```python
from build123d import *

# Parameters (mm, degrees)
SKETCH1_R           = 9.525
BOSS_EXTRUDE1_DEPTH = 3.175
SKETCH3_R           = 0.508
CUT_EXTRUDE1_DEPTH  = 25.4
SKETCH6_W           = 1.016
SKETCH6_H           = 1.016
CUT_EXTRUDE2_DEPTH  = 7.366
SKETCH7_W           = 1.012612731
SKETCH7_H           = 1.016
CUT_EXTRUDE3_DEPTH  = 7.366
SKETCH4_R           = 0.508


with BuildPart() as part:
    # Sketch1 → Boss-Extrude1 (new body)
    with BuildSketch(Plane(origin=(0, 0, 0), x_dir=(1, 0, 0), z_dir=(0, 1, 0))):
        Circle(SKETCH1_R)
    extrude(amount=BOSS_EXTRUDE1_DEPTH)

    # Sketch3 → Cut-Extrude1 (cut, symmetric)
    with BuildSketch(Plane.XY):
        with Locations((-8.509, 1.5875)):
            Circle(SKETCH3_R)
    extrude(amount=CUT_EXTRUDE1_DEPTH, both=True, mode=Mode.SUBTRACT)

    # Sketch6 → Cut-Extrude2 (cut)
    with BuildSketch(Plane.XY.offset(-7.62)):
        with Locations((-9.017, 1.5875)):
            Rectangle(SKETCH6_W, SKETCH6_H)
    extrude(amount=CUT_EXTRUDE2_DEPTH, mode=Mode.SUBTRACT)

    # Sketch7 → Cut-Extrude3 (cut)
    with BuildSketch(Plane.XY.offset(7.62)):
        with Locations((-9.015306366, 1.5875)):
            Rectangle(SKETCH7_W, SKETCH7_H)
    extrude(amount=-CUT_EXTRUDE3_DEPTH, mode=Mode.SUBTRACT)

    # Cut-Sweep1: sweep along a path in Sketch5
    with BuildLine(Plane(origin=(0, 0, 0), x_dir=(1, 0, 0), z_dir=(0, 1, 0))) as cut_sweep1_path:
        ThreePointArc((-7.554809844, -0.994609585), (7.62, 0), (-7.554809844, 0.994609585))
    # Sketch4 → Cut-Sweep1 (sweep, cut)
    with BuildSketch(Plane.XY):
        with Locations((9.525, 1.5875)):
            Circle(SKETCH4_R)
    sweep(path=cut_sweep1_path.line, mode=Mode.SUBTRACT)


solid = part.part
```
The model under review builds one solid part; all positions refer to its coordinate system, in mm. A direction names the side the tool comes from. Round coordinates to 2 decimals unless told otherwise and drop trailing zeros. Loops run counter-clockwise (first coordinate to the right, second up) from the corner with the lowest first, then second, coordinate; pieces in that order, holes last. Notation, with made-up numbers: M 61,24 L 95,24 A20 ccw 95,43 Z; hole C -12.5,-35 d5. An arc over 180 degrees is marked long. Put each result on its own line as item: value.
Q1. Consider section B-B, the plane y = 2.4. Give the boundary of the cut face in (x, z) (3 decimals), then the cut area to 3 significant figures.
Result set:
outline: C 0,0 d19.05
area: 285 mm²
Q2. Machinability: for faces 4 (the flat face through (-9, 2.096, -2)), 5 (the cylindrical face through (-8.04, 1.39, 0.06)), 6 (the flat face through (-9, 1.08, 2)), which of the approach directions +Z, -Z, +X, -X, +Y, -Y give a long, thin tool a straight path to every point of the face, cutting with its end or side? Answer none if there is none.
Result set:
face 4: -Z, -X
face 5: +Z, -Z
face 6: +Z, -X
Q3. Mouldability with a two-part tool opening along Y and no side actions: class faces 1 (the flat face through (-9, 2.096, 2)), 2 (the flat face through (0, 0, 0)), 3 (the flat face through (0, 3.175, 0)) as released by +Y, released by -Y, zero draft, split by the parting line, or undercut.
Result set:
face 1: undercut
face 2: released by -Y
face 3: released by +Y
Q4. For pin 1 (1.6 mm diameter, centred on x = -8.51, y = 1.59, fed in from +Z); pin 2 (4 mm diameter, centred on x = 0, z = -3.5, fed in from -Y); pin 3 (1 mm diameter, centred on y = 0.5, z = 1, fed in from -X), all flat-tipped, find the tip position at first contact; note any pin that passes through.
Result set:
pin 1: stops at z = 5.34
pin 2: stops at y = 0
pin 3: stops at x = -9.51
Q5. To check wall thickness, follow L1, parallel to X at y = 2.6, z = 2.5; L2, parallel to Z at x = -2.75, y = 1.7; L3, parallel to Z at x = 2, y = 1.6. State the ranges of each line that lie inside material, in increasing order.
Result set:
L1: x = -9.19 to 9.19
L2: z = -8.6 to 8.6
L3: z = -8.79 to 8.79
Q6. Consider section A-A, the plane z = 0. Give the boundary of the cut face in (x, y) (1 decimal), then the cut area to 3 significant figures.
Result set:
outline: M -9.5,0 L 9.5,0 L 9.5,1.1 A0.5 cw 9.5,2.1 L 9.5,3.2 L -9.5,3.2 Z; hole C -8.5,1.6 d1
area: 59.3 mm²
